from build123d import *

# Parameters (mm, degrees)
F0_W     = 75
F0_H     = 20
F0_R     = 3
F0_R_2   = 2.5
F0_R_3   = 2
F1_DEPTH = 30
F2_DEPTH = 5
F3_R     = 5
F4_SIZE  = 1


with BuildPart() as f1:
    # F0 (on Top) → F1 (new body)
    with BuildSketch(Plane.XY):
        Rectangle(F0_W, F0_H)
        with Locations((-26.8, 0)):
            Circle(F0_R, mode=Mode.SUBTRACT)
        with Locations((-16.1, 0)):
            Circle(F0_R_2, mode=Mode.SUBTRACT)
        with Locations((-5.4, 0)):
            Circle(F0_R_3, mode=Mode.SUBTRACT)
        with Locations((5.3, 0)):
            Circle(F0_R_3, mode=Mode.SUBTRACT)
        with Locations((16, 0)):
            Circle(F0_R_3, mode=Mode.SUBTRACT)
        with Locations((26.7, 0)):
            Circle(F0_R_3, mode=Mode.SUBTRACT)
    extrude(amount=F1_DEPTH)

    # F0 (on Top) → F2 (join)
    with BuildSketch(Plane.XY):
        with Locations((-26.8, 0)):
            Circle(F0_R)
        with Locations((-16.1, 0)):
            Circle(F0_R_2)
        with Locations((-5.4, 0)):
            Circle(F0_R_3)
        with Locations((5.3, 0)):
            Circle(F0_R_3)
        with Locations((16, 0)):
            Circle(F0_R_3)
        with Locations((26.7, 0)):
            Circle(F0_R_3)
    extrude(amount=F2_DEPTH)

    # F3
    f3_edges = [f1.edges().sort_by_distance(p)[0] for p in [
        (37.5, -10, 15),
        (37.5, 10, 15),
        (-37.5, -10, 15),
        (-37.5, 10, 15),
    ]]
    fillet(f3_edges, radius=F3_R)

    # F4
    f4_edges = [f1.edges().sort_by_distance(p)[0] for p in [
        (-29.8, 0, 30),
        (-18.6, 0, 30),
        (-7.4, 0, 30),
        (3.3, 0, 30),
        (14, 0, 30),
        (24.7, 0, 30),
        (0, -10, 30),
    ]]
    chamfer(f4_edges, length=F4_SIZE)


solid = f1.part
The model under review builds one solid part; all positions refer to its coordinate system, in mm. A direction names the side the tool comes from. Give positions to 0.01 mm unless a question says otherwise; leave off trailing zeros. Order: outer loops, then holes, each group sorted by start corner. A loop starts at its lowest first (then second) coordinate and runs counter-clockwise, first axis right, second up. Notation, with made-up numbers: M -34.75,59 L -20.75,59 A29 cw -20.75,85 Z; hole C 57.25,6 d2. An arc over 180 degrees is marked long. Use one line per item in the form item = value. Start each with the question number.
Item 1: We need section B-B on x = -16.1. Give the boundary of the cut face in (y, z).
Item 2: To check wall thickness, follow line 1 along Y through (x, z) = (-26.8, 22.75); line 2 along Y through (x, z) = (16, 14); line 3 along Z through (x, y) = (-30, -1). State the ranges of each line that lie inside material, in increasing order. Write a range as from..to.
Item 3: Insertion check: pin 1 Ø2 at (x, y) = (-23, 3) entering from -Z; pin 2 Ø5 at (x, y) = (26.7, 0) entering from +Z; pin 3 Ø3 at (x, y) = (-26, -0.5) entering from +Z; pin 4 Ø2 at (x, y) = (15.5, 1) entering from +Z. Each pin has a flat end and moves straight along its axis. Give the tip position at first contact, or say it passes through.
Item 4: For faces 1 (the cylindrical face through (-36.07, -8.5, 14.7)), 2 (the flat face through (16, 0, 5)), list the 3-axis set-ups (+Z, -Z, +X, -X, +Y, -Y) from which the entire face can be reached by the end or side of a thin tool; tool diameter is ignored.
Item 5: We need section C-C on x = -26.8. Give the boundary of the cut face in (y, z).
Item 6: We need section A-A on z = 20.75. Give the boundary of the cut face in (x, y), plus the area to 3 significant figures.
Completed:
q1.outline = M -10,0 L 10,0 L 10,29 L 9,30 L 3.5,30 L 2.5,29 L 2.5,5 L -2.5,5 L -2.5,29 L -3.5,30 L -9,30 L -10,29 Z
q2.line_1 = -10..-3, 3..10
q2.line_2 = -10..-2, 2..10
q2.line_3 = 0..29.35
q3.pin_1 = 0
q3.pin_2 = 29.5
q3.pin_3 = 5
q3.pin_4 = 29.12
q4.face_1 = +Z, -Z, -X, -Y
q4.face_2 = +Z
q5.outline = M -10,0 L 10,0 L 10,29 L 9,30 L 4,30 L 3,29 L 3,5 L -3,5 L -3,29 L -4,30 L -9,30 L -10,29 Z
q6.outline = M -37.5,-5 A5 ccw -32.5,-10 L 32.5,-10 A5 ccw 37.5,-5 L 37.5,5 A5 ccw 32.5,10 L -32.5,10 A5 ccw -37.5,5 Z; hole C -26.8,0 d6; hole C -16.1,0 d5; hole C -5.4,0 d4; hole C 5.3,0 d4; hole C 16,0 d4; hole C 26.7,0 d4
q6.area = 1,380 mm²
